The model under review builds one solid part; all positions refer to its coordinate system, in mm. A direction names the side the tool comes from. Round coordinates to 2 decimals unless told otherwise and drop trailing zeros. Order: outer loops, then holes, each group sorted by start corner. A loop starts at its lowest first (then second) coordinate and runs counter-clockwise, first axis right, second up. Notation, with made-up numbers: M 55.25,42.25 L 88.25,42.25 A29 ccw 88.25,73.25 Z; hole C 86,87 d6. An arc over 180 degrees is marked long. Use a Markdown table: item, result. Add a question column.
1. Consider section C-C on x = 12. State the section outline as (y, z) points, then the cut area to 3 significant figures.
2. Insertion check: P1, Ø7.5, axis at x = 10.5, y = -37.5, coming from the +Z side; P2, Ø6, axis at y = -10, z = -14.5, coming from the -X side; P3, Ø14.5, axis at x = -6, z = -41.5, coming from the +Y side; P4, Ø8, axis at x = -20, z = -10, coming from the -Y side. Each pin has a flat end and moves straight along its axis. Give the tip position at first contact, or say it passes through.
3. Consider section A-A on y = 6.5. State the section outline as (x, z) points.
4. Consider section D-D on y = -9.5. State the section outline as (x, z) points, then the cut area to 3 significant figures.
5. For faces 1 (the flat face through (6.8, -52.8, -75)), 2 (the cylindrical face through (14.73, -23.93, -76.5)), 3 (the cylindrical face through (4.867, -19.629, -82.482)), 4 (the flat face through (29, 5, 0)), list the 3-axis set-ups (+Z, -Z, +X, -X, +Y, -Y) from which the entire face can be reached by the end or side of a thin tool; tool diameter is ignored.
6. Consider section B-B on z = -56. State the section outline as (x, y) points, then the cut area to 3 significant figures.
7. To check wall thickness, follow probe 1 along X at (y, z) = (-52, -81); probe 2 along Y at (x, z) = (-2, -61.5); probe 3 along Z at (x, y) = (-2.5, 4.5). State the ranges of each line that lie inside material, in increasing order.
from build123d import *

# Parameters (mm, degrees)
IZIM1_W                     = 69
IZIM1_H                     = 45
IZIM1_R                     = 8
Y_KSEKLIK_EKSTR_ZYON1_DEPTH = 10
Y_KSEKLIK_EKSTR_ZYON2_DEPTH = 69
RADYUS1_R                   = 5
KES_EKSTR_ZYON2_DEPTH       = 57
IZIM6_R                     = 19
Y_KSEKLIK_EKSTR_ZYON3_DEPTH = 10
Y_KSEKLIK_EKSTR_ZYON4_START = 3
IZIM7_R                     = 19
Y_KSEKLIK_EKSTR_ZYON4_DEPTH = 3
Y_KSEKLIK_EKSTR_ZYON5_DEPTH = 10
KES_EKSTR_ZYON3_REACH       = 137.656
IZIM10_R                    = 8
RADYUS3_R                   = 25
RADYUS4_R                   = 25


with BuildPart() as part:
    # Çizim1 → Yükseklik-Ekstrüzyon1 (new body)
    with BuildSketch(Plane.XY):
        Rectangle(IZIM1_W, IZIM1_H)
        with Locations((-12.5, 4.5)):
            Circle(IZIM1_R, mode=Mode.SUBTRACT)
    extrude(amount=Y_KSEKLIK_EKSTR_ZYON1_DEPTH)

    # Çizim2 → Yükseklik-Ekstrüzyon2 (add)
    with BuildSketch(Plane(origin=(34.5, 0, 0), x_dir=(0, 0, -1), z_dir=(1, 0, 0))):
        Polygon((0, -12.5), (90, -12.5), (90, -52.5), (78, -52.5), (78, -22.5), (0, -22.5), align=None)
    extrude(amount=-Y_KSEKLIK_EKSTR_ZYON2_DEPTH)

    # Radyus1
    radyus1_edges = [part.edges().sort_by_distance(p)[0] for p in [
        (0, -22.5, -78),
    ]]
    fillet(radyus1_edges, radius=RADYUS1_R)

    # Çizim4 → Kes-Ekstrüzyon2 (cut)
    with BuildSketch(Plane(origin=(0, -12.5, 0), x_dir=(1, 0, 0), z_dir=(0, 1, 0))):
        with BuildLine():
            ThreePointArc((-34.5, 0), (-13.286796564, 8.786796564), (-4.5, 30))
            Line((-4.5, 30), (-4.5, 90))
            Line((-4.5, 90), (-34.5, 90))
            Line((-34.5, 90), (-34.5, 0))
        make_face()
        with BuildLine():
            ThreePointArc((-62.385076525, 41.064470488), (-59.318683634, 13.146723088), (-34.5, 0))
            Line((-34.5, 0), (-34.5, 90))
            Line((-34.5, 90), (-58.233748988, 48.34963648))
            Line((-58.233748988, 48.34963648), (-62.385076525, 41.064470488))
        make_face()
    extrude(amount=-KES_EKSTR_ZYON2_DEPTH, mode=Mode.SUBTRACT)

    # Çizim6 → Yükseklik-Ekstrüzyon3 (add)
    with BuildSketch(Plane(origin=(0, 0, -90), x_dir=(-1, 0, 0), z_dir=(0, 0, -1))):
        with Locations((-15, -52.5)):
            Circle(IZIM6_R)
    extrude(amount=Y_KSEKLIK_EKSTR_ZYON3_DEPTH)

    # Çizim7 → Yükseklik-Ekstrüzyon4 (add)
    with BuildSketch(Plane.XY.offset(-78).offset(Y_KSEKLIK_EKSTR_ZYON4_START)):
        with Locations(Location((15, -52.5, 0), (0, 0, 180))):
            Circle(IZIM7_R)
    extrude(amount=-Y_KSEKLIK_EKSTR_ZYON4_DEPTH)

    # loft from a face of the part (loft1)
    loft([part.faces().sort_by_distance((15, -60.56385045, -90))[0], part.faces().sort_by_distance((15, -60.56385045, -78))[0]])

    # Çizim15 → Yükseklik-Ekstrüzyon5 (add)
    with BuildSketch(Plane(origin=(24.5, 0, 0), x_dir=(0, 0, -1), z_dir=(1, 0, 0))):
        with BuildLine():
            Line((0, 22.5), (0, -12.5))
            Line((0, -12.5), (90, -12.5))
            Line((90, -12.5), (90, -52.5))
            Line((90, -52.5), (98, -52.5))
            Line((98, -52.5), (98, -46.937300736))
            Line((98, -46.937300736), (98, -2.5))
            Line((98, -2.5), (25, -2.5))
            ThreePointArc((25, -2.5), (7.32233047, 4.82233047), (0, 22.5))
        make_face()
    extrude(amount=-Y_KSEKLIK_EKSTR_ZYON5_DEPTH)

    # Çizim10 → Kes-Ekstrüzyon3 (cut, up to next)
    with BuildSketch(Plane(origin=(0, 0, -100), x_dir=(-1, 0, 0), z_dir=(0, 0, -1)), mode=Mode.PRIVATE) as kes_ekstr_zyon3_sk1:
        with Locations((-15, -52.5)):
            Circle(IZIM10_R)
    kes_ekstr_zyon3_tool1 = extrude(kes_ekstr_zyon3_sk1.sketch, amount=-KES_EKSTR_ZYON3_REACH, mode=Mode.PRIVATE) & part.part
    add(kes_ekstr_zyon3_tool1.solids().sort_by_distance((15, -52.5, -100))[0], mode=Mode.SUBTRACT)

    # Radyus3
    radyus3_edges = [part.edges().sort_by_distance(p)[0] for p in [
        (19.5, -2.5, -98),
    ]]
    fillet(radyus3_edges, radius=RADYUS3_R)

    # Radyus4
    radyus4_edges = [part.edges().sort_by_distance(p)[0] for p in [
        (29.5, -12.5, -90),
        (5, -12.5, -90),
    ]]
    fillet(radyus4_edges, radius=RADYUS4_R)


solid = part.part
Answer block:
| question | item | result |
|---|---|---|
| 1 | outline | M -71.26,-100 L -59.92,-100 L -59.92,-75 L -71.26,-75 Z; M -45.08,-100 L -33.74,-100 L -33.74,-89.72 A25 ccw -12.5,-65 L -12.5,0 L 22.5,0 L 22.5,10 L -22.5,10 L -22.5,-73 A5 cw -27.5,-78 L -33.74,-78 L -33.74,-75 L -45.08,-75 Z |
| 1 | area | 1,920 mm^2 |
| 2 | P1 | z = -75 |
| 2 | P2 | x = -9.89 |
| 2 | P3 | y = -12.5 |
| 2 | P4 | through |
| 3 | outline | M -34.5,0 L -20.25,0 L -20.25,10 L -34.5,10 Z; M -4.75,0 L 14.5,0 L 14.5,-5.79 L 24.5,-5.79 L 24.5,0 L 34.5,0 L 34.5,10 L -4.75,10 Z |
| 4 | outline | M -34.5,0 L 14.5,0 L 14.5,-90.35 L 24.5,-90.35 L 24.5,0 L 34.5,0 L 34.5,10 L -34.5,10 Z |
| 4 | area | 1,590 mm^2 |
| 5 | face 1 | +Z, +X, -X, -Y |
| 5 | face 2 | +Z, +X, -X |
| 5 | face 3 | -Z, -X, +Y |
| 5 | face 4 | -Z, +X, +Y |
| 6 | outline | M -4.5,-22.5 L 34.5,-22.5 L 34.5,-12.5 L 24.5,-12.5 L 24.5,-2.5 L 14.5,-2.5 L 14.5,-12.5 L -4.5,-12.5 Z |
| 6 | area | 490 mm^2 |
| 7 | probe 1 | -4.5 to 7.02, 22.98 to 34.5 |
| 7 | probe 2 | -22.5 to -12.5 |
| 7 | probe 3 | 0 to 10 |
